Design review of the part shown in the three views and the two pictorial views. Dimensions are in mm from the part's minimum x, y and z. A direction names the side the tool comes from. Give positions to 0.01 mm unless a question says otherwise; leave off trailing zeros. Loops run counter-clockwise (first coordinate to the right, second up) from the corner with the lowest first, then second, coordinate; pieces in that order, holes last.
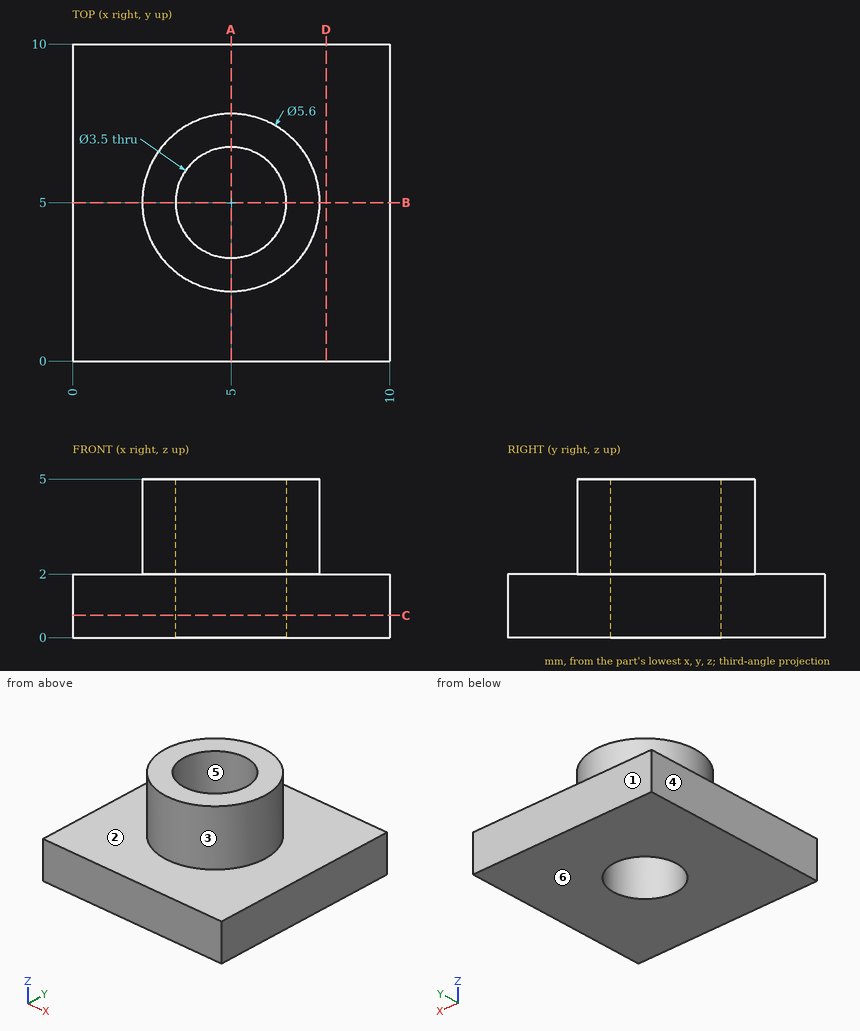
Q1. For pin 1 Ø1.5 at (y, z) = (1.5, 2) entering from -X; pin 2 Ø3 at (x, y) = (5, 5) entering from +Z; pin 3 Ø3 at (x, z) = (7.5, 4) entering from -Y, all flat-tipped, find the tip position at first contact; note any pin that passes through.
Answers:
pin 1: stops at x = 0
pin 2: passes through
pin 3: stops at y = 2.38
Q2. For probe 1 along Y at (x, z) = (5, 1.7); probe 2 along Y at (x, z) = (5, 2.45); probe 3 along X at (y, z) = (5.75, 2.05), list the stretches that pass through material, from the lowest coordinate up.
Answers:
probe 1: y = 0 to 3.25, 6.75 to 10
probe 2: y = 2.2 to 3.25, 6.75 to 7.8
probe 3: x = 2.3 to 3.42, 6.58 to 7.7
Q3. Consider section D-D on x = 8. Give the boundary of the cut face in (y, z), plus the area to 3 significant figures.
Answers:
outline: (0, 0) - (10, 0) - (10, 2) - (0, 2) - close
area: 20.0 mm2
Q4. Consider section C-C on z = 0.7. Give the boundary of the cut face in (x, y), plus the area to 3 significant figures.
Answers:
outline: (0, 0) - (10, 0) - (10, 10) - (0, 10) - close; hole circle Ø3.5 at (5, 5)
area: 90.4 mm2
Q5. Mouldability with a two-part tool opening along X and no side actions: class the marked faces 3, 4, 5 and 6 as +X half, -X half, draft (parallel to the pull), parting line (faces both ways), or undercut.
Answers:
face 3: parting line
face 4: -X half
face 5: undercut
face 6: draft
Q6. Consider section A-A on x = 5. Give the boundary of the cut face in (y, z), plus the area to 3 significant figures.
Answers:
outline: (0, 0) - (3.25, 0) - (3.25, 5) - (2.2, 5) - (2.2, 2) - (0, 2) - close; (6.75, 0) - (10, 0) - (10, 2) - (7.8, 2) - (7.8, 5) - (6.75, 5) - close
area: 19.3 mm2
Q7. Machinability: for the marked faces 1 and 2, which of the approach directions +Z, -Z, +X, -X, +Y, -Y give a long, thin tool a straight path to every point of the face, cutting with its end or side? Answer none if there is none.
Answers:
face 1: +Z, -Z, +X, -X, +Y
face 2: +Z
